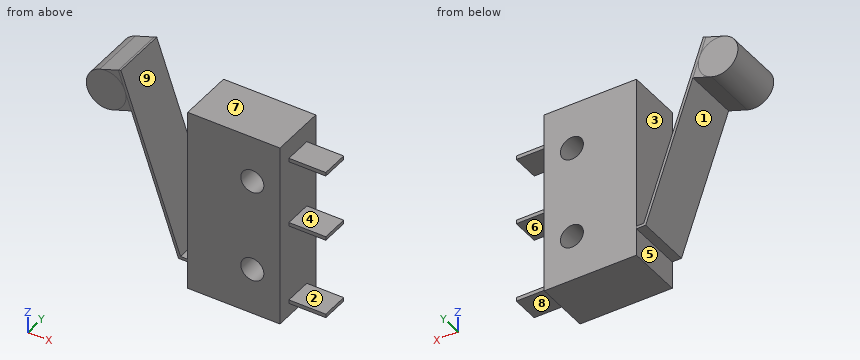
Autodesk Inventor part; units mm, degrees
ref_plane "YZ Plane" through (0, 0, 0) normal (1, 0, 0) x (0, 1, 0)
ref_plane "XZ Plane" through (0, 0, 0) normal (0, 1, 0) x (-1, 0, 0)
ref_plane "XY Plane" through (0, 0, 0) normal (0, 0, 1) x (1, 0, 0)
sketch "Sketch1" plane through (0, 0, 0) normal (0, 1, 0) x (-1, 0, 0)
  line L0 (0, 0) -> (10, 0)
  line L1 (10, 0) -> (10, -20)
  line L2 (10, -20) -> (0, -20)
  line L3 (0, -20) -> (0, 0)
  circle A0 centre (3, -5) radius 1.25
  circle A1 centre (3, -15) radius 1.25
  dimension "d0" = 10
  dimension "d1" = 20
  dimension "d2" = 2.5
  dimension "d3" = 2.5
  dimension "d4" = 3
  dimension "d5" = 3
  dimension "d6" = 5
  dimension "d7" = 5
extrude "Extrusion1" add sketch "Sketch1" along normal blind 6
sketch "Sketch2" plane through (0, 6, 0) normal (0, 1, 0) x (1, 0, 0)
  line L0 (0, 20) -> (-10, 20)
  line L1 (-10, 20) -> (-10, 0)
  line L2 (-10, 0) -> (0, 0)
  line L3 (0, 0) -> (0, 20)
  circle A0 centre (-3, 15) radius 1.25
  circle A1 centre (-3, 5) radius 1.25
  circle A2 centre (-18.85, 1) radius 2.15
  line L4 (-10, 20) -> (-10, 0)
  line L5 (-10, 17) -> (-11, 17)
  line L6 (-11, 17) -> (-17.5269, -1.7376)
  line L7 (-16.1124, 2.3231) -> (-18.1428, 3.0303)
  line L8 (-19.5572, -1.0303) -> (-17.2436, -1.8363)
  line L9 (-17.2436, -1.8363) -> (-10.7868, 16.7)
  line L10 (-10.7868, 16.7) -> (-10, 16.7)
  dimension "d10" = 4.3
  dimension "d11" = 18.85
  dimension "d12" = 1
  dimension "d13" = 1
  dimension "d15" = 3
  dimension "d16" = 0.3
  dimension "d17" = 0.3
extrude "Extrusion2" add sketch "Sketch2" against normal blind 6 contours L1 L10 L9 L8 L6 L5 | L6 A2 L7 | L6 L8 A2 | A2
sketch "Sketch3" plane through (0, 0, 0) normal (1, 0, 0) x (0, 0, -1)
  line L0 (2.1, 4.5) -> (2.5, 4.5)
  line L1 (2.5, 4.5) -> (2.5, 1.5)
  line L2 (2.5, 1.5) -> (2.1, 1.5)
  line L3 (2.1, 1.5) -> (2.1, 4.5)
  line L4 (0, 0) -> (20, 0)
  line L5 (20, 0) -> (20, 6)
  line L6 (0, 6) -> (20, 6)
  line L7 (0, 0) -> (0, 6)
  line L8 (9.4, 4.5) -> (9.8, 4.5)
  line L9 (9.8, 4.5) -> (9.8, 1.5)
  line L10 (9.8, 1.5) -> (9.4, 1.5)
  line L11 (9.4, 1.5) -> (9.4, 4.5)
  line L12 (18.2, 4.5) -> (18.6, 4.5)
  line L13 (18.6, 4.5) -> (18.6, 1.5)
  line L14 (18.6, 1.5) -> (18.2, 1.5)
  line L15 (18.2, 1.5) -> (18.2, 4.5)
  dimension "d20" = 3
  dimension "d21" = 3
  dimension "d22" = 3
  dimension "d23" = 0.4
  dimension "d24" = 0.4
  dimension "d25" = 0.4
  dimension "d26" = 1.5
  dimension "d27" = 1.5
  dimension "d28" = 2.5
  dimension "d29" = 7.7
  dimension "d31" = 16.5
extrude "Extrusion3" add sketch "Sketch3" along normal blind 4 contours L0 L1 L2 L3 | L8 L9 L10 L11 | L12 L13 L14 L15
equation "\"d21\" = d20"
equation "\"d22\" = d21"
equation "\"d24\" = d23"
equation "\"d25\" = d23"
equation "\"d27\" = d26"
properties part number "LimitSwitch"
The model under review builds one solid part; all positions refer to its coordinate system, in mm. Face numbers are marked on the shaded views. A direction names the side the tool comes from. Coordinates: 2 decimals unless noted, no trailing zeros. Order: outer loops, then holes, each group sorted by start corner. A loop starts at its lowest first (then second) coordinate and runs counter-clockwise, first axis right, second up. Notation, with made-up numbers: (32.25, 61) -> (86.25, 61) arc R19 ccw to (86.25, 78) -> close; hole circle Ø6 at (1, -32.5). An arc over 180 degrees is marked (long way). Answer in a Markdown table with one row per item.
(1) Consider section A-A (x = -3). Write out the cut boundary in (y, z), plus the area to 3 significant figures.
Answers:
| item | result |
|---|---|
| outline | (0, -20) -> (6, -20) -> (6, -16.25) -> (0, -16.25) -> close; (0, -13.75) -> (6, -13.75) -> (6, -6.25) -> (0, -6.25) -> close; (0, -3.75) -> (6, -3.75) -> (6, 0) -> (0, 0) -> close |
| area | 90.0 mm² |
(2) The part is to be moulded in two halves that separate along Z. For the marked faces 1, 2, 3 and 4, say which applies: +Z half, -Z half, draft (parallel to the pull), parting line (faces both ways), or undercut.
Answers:
| item | result |
|---|---|
| face 1 | -Z half |
| face 2 | undercut |
| face 3 | draft |
| face 4 | undercut |
(3) Insertion check: pin 1 (0.9 mm diameter, centred on x = 2, y = 2.5, fed in from +Z); pin 2 (1 mm diameter, centred on y = 5, z = -11.5, fed in from +X); pin 3 (2.5 mm diameter, centred on y = 4, z = -18.5, fed in from -X). Each pin has a flat end and moves straight along its axis. Give the tip position at first contact, or say it passes through.
Answers:
| item | result |
|---|---|
| pin 1 | z = -2.1 |
| pin 2 | x = 0 |
| pin 3 | x = -10 |
(4) Consider section C-C (z = -7.5). Write out the cut boundary in (x, y), plus the area to 3 significant figures.
Answers:
| item | result |
|---|---|
| outline | (-14.31, 0) -> (-13.99, 0) -> (-13.99, 6) -> (-14.31, 6) -> close; (-10, 0) -> (0, 0) -> (0, 6) -> (-10, 6) -> close |
| area | 61.9 mm² |
(5) Wall thickness on line 1 along Z through (x, y) = (-3, 1.2); line 2 along X through (y, z) = (2.4, -1); line 3 along Z through (x, y) = (-9.25, 2.9): over which ranges is each line inside the solid? List them lowest first.
Answers:
| item | result |
|---|---|
| line 1 | -20 to -16.25, -13.75 to -6.25, -3.75 to 0 |
| line 2 | -21 to -16.26, -10 to 0 |
| line 3 | -20 to 0 |
(6) Machinability: for the marked faces 5, 6, 7, 8 and 9, which of the approach directions +Z, -Z, +X, -X, +Y, -Y give a long, thin tool a straight path to every point of the face, cutting with its end or side? Answer none if there is none.
Answers:
| item | result |
|---|---|
| face 5 | -Z, -X, +Y, -Y |
| face 6 | +X, +Y, -Y |
| face 7 | +Z, +X, +Y, -Y |
| face 8 | -Z, +X, +Y, -Y |
| face 9 | +Z, +Y, -Y |
(7) Consider section D-D (z = -5). Write out the cut boundary in (x, y), plus the area to 3 significant figures.
Answers:
| item | result |
|---|---|
| outline | (-15.18, 0) -> (-14.86, 0) -> (-14.86, 6) -> (-15.18, 6) -> close; (-10, 0) -> (-4.25, 0) -> (-4.25, 6) -> (-10, 6) -> close; (-1.75, 0) -> (0, 0) -> (0, 6) -> (-1.75, 6) -> close |
| area | 46.9 mm² |
(8) Consider section B-B (y = 0.55). Write out the cut boundary in (x, z).
Answers:
| item | result |
|---|---|
| outline | (-19.56, 1.03) arc R2.15 ccw to (-18.14, -3.03) -> (-16.11, -2.32) -> (-11, -17) -> (-10, -17) -> (-10, -20) -> (0, -20) -> (0, 0) -> (-10, 0) -> (-10, -16.7) -> (-10.79, -16.7) -> (-17.24, 1.84) -> close; hole circle Ø2.5 at (-3, -15); hole circle Ø2.5 at (-3, -5) |
